Geometry check sheet. Reference: the model listing, model coordinates, mm. Face numbers are marked on the shaded views. A direction names the side the tool comes from. Round coordinates to 2 decimals unless told otherwise and drop trailing zeros. Write each loop counter-clockwise with the first axis right and the second up, starting at its lowest first coordinate (ties: lowest second). Pieces come first, ordered by that corner, then holes. Notation, with made-up numbers: (-30, -34) -> (3, -34) arc R11 ccw to (3, -21) -> close; hole circle Ø3 at (24.25, 7). An arc over 180 degrees is marked (long way). Use a Markdown table: item, result.
```python
from build123d import *

# Parameters (mm, degrees)
ODGI_CIE_BAZOWE1_DEPTH      = 40
SZCZELINA_POD_RUB_M52_DEPTH = 2
OTW_R_POD_RUB_M81_D         = 9
SZKIC10_W                   = 12.5
SZKIC10_H                   = 15
WYTNIJ_WYCI_GNI_CIE1_DEPTH  = 79.89866919
ZAOKR_GLENIE1_R             = 5


# Read off the part's stored shape, not the designer's step: Szczelina pod śrubę M52
# Sheet-metal steps are written as plain solids
with BuildPart() as part:
    # Szkic1 → Odgięcie bazowe1 (new, symmetric)
    with BuildSketch(Plane(origin=(0, 0, 0), x_dir=(0, 0, -1), z_dir=(1, 0, 0))):
        with BuildLine():
            Line((27.5, 40), (27.5, 5))
            ThreePointArc((27.5, 5), (26.035533906, 1.464466094), (22.5, 0))
            Line((22.5, 0), (-22.5, 0))
            ThreePointArc((-22.5, 0), (-26.035533906, 1.464466094), (-27.5, 5))
            Line((-27.5, 5), (-27.5, 40))
            Line((-27.5, 40), (-25.5, 40))
            Line((-25.5, 40), (-25.5, 5))
            ThreePointArc((-25.5, 5), (-24.621320344, 2.878679656), (-22.5, 2))
            Line((-22.5, 2), (22.5, 2))
            ThreePointArc((22.5, 2), (24.621320344, 2.878679656), (25.5, 5))
            Line((25.5, 5), (25.5, 40))
            Line((25.5, 40), (27.5, 40))
        make_face()
    extrude(amount=ODGI_CIE_BAZOWE1_DEPTH, both=True)

    # Szczelina pod śrubę M52 outline → Szczelina pod śrubę M52 (cut)
    with BuildSketch(Plane(origin=(0, 0, 0), x_dir=(1, 0, 0), z_dir=(0, 1, 0))):
        with BuildLine():
            ThreePointArc((5, -12.25), (2.25, -15), (5, -17.75))
            Line((5, -17.75), (20, -17.75))
            ThreePointArc((20, -17.75), (22.75, -15), (20, -12.25))
            Line((20, -12.25), (5, -12.25))
        make_face()
        with BuildLine():
            ThreePointArc((-20, -12.25), (-22.75, -15), (-20, -17.75))
            Line((-20, -17.75), (-5, -17.75))
            ThreePointArc((-5, -17.75), (-2.25, -15), (-5, -12.25))
            Line((-5, -12.25), (-20, -12.25))
        make_face()
        with BuildLine():
            ThreePointArc((-5, 12.25), (-2.25, 15), (-5, 17.75))
            Line((-5, 17.75), (-20, 17.75))
            ThreePointArc((-20, 17.75), (-22.75, 15), (-20, 12.25))
            Line((-20, 12.25), (-5, 12.25))
        make_face()
        with BuildLine():
            ThreePointArc((20, 12.25), (22.75, 15), (20, 17.75))
            Line((20, 17.75), (5, 17.75))
            ThreePointArc((5, 17.75), (2.25, 15), (5, 12.25))
            Line((5, 12.25), (20, 12.25))
        make_face()
    extrude(amount=SZCZELINA_POD_RUB_M52_DEPTH, mode=Mode.SUBTRACT)

    # Otwór pod śrubę M81 (through all)
    with Locations(Plane(origin=(0, 0, -27.5), x_dir=(-1, 0, 0), z_dir=(0, 0, -1))):
        with Locations((-27.5, 28), (27.5, 28)):
            Hole(OTW_R_POD_RUB_M81_D / 2)

    # Szkic10 → Wytnij-wyciągnięcie1 (cut, through all)
    with BuildSketch(Plane(origin=(0, 0, -27.5), x_dir=(-1, 0, 0), z_dir=(0, 0, -1))):
        with Locations((-33.75, 7.5)):
            Rectangle(SZKIC10_W, SZKIC10_H)
        with Locations((33.75, 7.5)):
            Rectangle(SZKIC10_W, SZKIC10_H)
    extrude(amount=-WYTNIJ_WYCI_GNI_CIE1_DEPTH, mode=Mode.SUBTRACT)

    # Zaokrąglenie1
    zaokr_glenie1_edges = [part.edges().sort_by_distance(p)[0] for p in [
        (-40, 40, -26.5),
        (-40, 40, 26.5),
        (40, 15, -26.5),
        (40, 15, 26.5),
        (-40, 15, -26.5),
        (-40, 15, 26.5),
        (40, 40, -26.5),
        (40, 40, 26.5),
    ]]
    fillet(zaokr_glenie1_edges, radius=ZAOKR_GLENIE1_R)


solid = part.part
```
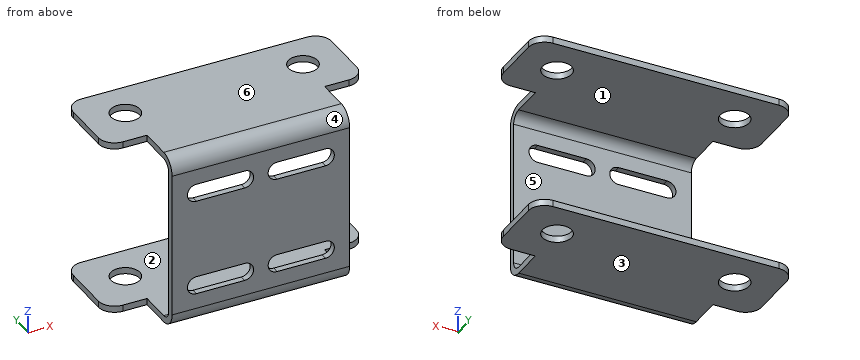
(1) Thickness scan on line 1 (Z direction, x = -20, y = 30); line 2 (Y direction, x = -5, z = 22.5); line 3 (Z direction, x = -21, y = 4). Record the ranges inside material, lowest first.
A:
| item | result |
|---|---|
| line 1 | z = -27.5 to -25.5, 25.5 to 27.5 |
| line 2 | y = 0 to 2 |
| line 3 | z = -27.4 to -25.33, 25.33 to 27.4 |
(2) Section check D-D on x = -24. Record the cut outline in (y, z), plus the area to 3 significant figures.
A:
| item | result |
|---|---|
| outline | (0, -22.5) arc R5 ccw to (5, -27.5) -> (25.17, -27.5) -> (25.17, -25.5) -> (5, -25.5) arc R3 cw to (2, -22.5) -> (2, 22.5) arc R3 cw to (5, 25.5) -> (25.17, 25.5) -> (25.17, 27.5) -> (5, 27.5) arc R5 ccw to (0, 22.5) -> close; (30.83, -27.5) -> (40, -27.5) -> (40, -25.5) -> (30.83, -25.5) -> close; (30.83, 25.5) -> (40, 25.5) -> (40, 27.5) -> (30.83, 27.5) -> close |
| area | 233 mm2 |
(3) Gauge pin test, flat ends, axial feed: pin 1 Ø0.6 at (x, y) = (12.5, 1.5) entering from -Z; pin 2 Ø6 at (x, z) = (29, -15) entering from -Y; pin 3 Ø2 at (x, z) = (32.5, -26.5) entering from -Y; pin 4 Ø1.6 at (x, y) = (-15.5, 1.5) entering from -Z. Record the tip position at first contact, or that the pin passes through.
A:
| item | result |
|---|---|
| pin 1 | stops at z = -26.34 |
| pin 2 | stops at y = 0 |
| pin 3 | stops at y = 15 |
| pin 4 | stops at z = -26.71 |
(4) Release check for a two-part mould opening along Z. For the marked faces 1, 2, 3 and 4 record: +Z half, -Z half, draft (parallel to the pull), parting line (faces both ways), or undercut.
A:
| item | result |
|---|---|
| face 1 | undercut |
| face 2 | undercut |
| face 3 | -Z half |
| face 4 | +Z half |
(5) Section check C-C on y = 31. Record the cut outline in (x, z).
A:
| item | result |
|---|---|
| outline | (-40, -27.5) -> (-30.85, -27.5) -> (-30.85, -25.5) -> (-40, -25.5) -> close; (-40, 25.5) -> (-30.85, 25.5) -> (-30.85, 27.5) -> (-40, 27.5) -> close; (-24.15, -27.5) -> (24.15, -27.5) -> (24.15, -25.5) -> (-24.15, -25.5) -> close; (-24.15, 25.5) -> (24.15, 25.5) -> (24.15, 27.5) -> (-24.15, 27.5) -> close; (30.85, -27.5) -> (40, -27.5) -> (40, -25.5) -> (30.85, -25.5) -> close; (30.85, 25.5) -> (40, 25.5) -> (40, 27.5) -> (30.85, 27.5) -> close |
(6) Access from +Z, -Z, +X, -X, +Y, -Y to the whole of each face (thin tool, end or side, straight path). Record for the marked faces 5 and 6.
A:
| item | result |
|---|---|
| face 5 | +X, -X, +Y |
| face 6 | +Z, +X, -X, +Y, -Y |
(7) Section check A-A on z = -15. Record the cut outline in (x, y).
A:
| item | result |
|---|---|
| outline | (-27.5, 0) -> (-22.75, 0) -> (-22.75, 2) -> (-27.5, 2) -> close; (-2.25, 0) -> (2.25, 0) -> (2.25, 2) -> (-2.25, 2) -> close; (22.75, 0) -> (27.5, 0) -> (27.5, 2) -> (22.75, 2) -> close |
(8) Section check B-B on x = -7.5. Record the cut outline in (y, z).
A:
| item | result |
|---|---|
| outline | (0, -22.5) arc R5 ccw to (5, -27.5) -> (40, -27.5) -> (40, -25.5) -> (5, -25.5) arc R3 cw to (2, -22.5) -> (2, -17.75) -> (0, -17.75) -> close; (0, -12.25) -> (2, -12.25) -> (2, 12.25) -> (0, 12.25) -> close; (0, 17.75) -> (2, 17.75) -> (2, 22.5) arc R3 cw to (5, 25.5) -> (40, 25.5) -> (40, 27.5) -> (5, 27.5) arc R5 ccw to (0, 22.5) -> close |
